Autodesk Inventor part; units mm, degrees
ref_plane "Arbeitsebene1" through (62.6214, -145.6709, 60.7697) normal (-1, 0, 0) x (0, -0.0042, 1)
ref_plane "YZ Plane" through (0, 0, 0) normal (1, 0, 0) x (0, 1, 0)
ref_plane "XZ Plane" through (0, 0, 0) normal (0, 1, 0) x (-1, 0, 0)
ref_plane "Arbeitsebene1" through (62.6214, -145.6709, 60.7697) normal (-1, 0, 0) x (0, -0.0042, 1)
sketch "Skizze1" plane through (62.6214, -145.6709, 60.7697) normal (-1, 0, 0) x (0, -0.0042, 1)
  circle A0 centre (0, 0) radius 10
  point P0 (-61.3791, 145.4152)
  dimension "d0" = 20
extrude "Extrusion1" add sketch "Skizze1" against normal blind 37
sketch "Skizze2" plane through (99.6214, -145.6709, 60.7697) normal (1, 0, 0) x (0, 0, -1)
  circle A0 centre (0, 0) radius 10
  circle A1 centre (0, 0) radius 12
  point P0 (60.7697, 145.6709)
  dimension "d3" = 24
extrude "Extrusion2" add sketch "Skizze2" along normal blind 83 contours A0 | A1
sketch "Skizze3" plane through (182.6214, -145.6709, 60.7697) normal (1, 0, 0) x (0, 0, -1)
  circle A0 centre (0, 0) radius 12
  circle A1 centre (0, 0) radius 14
  point P0 (60.7697, 145.6709)
  dimension "d6" = 28
extrude "Extrusion3" add sketch "Skizze3" along normal blind 191 contours A0 | A1
sketch "Skizze4" plane through (373.6214, -145.6709, 60.7697) normal (1, 0, 0) x (0, 0, -1)
  circle A0 centre (0, 0) radius 10
  circle A1 centre (0, 0) radius 12
  point P0 (60.7697, 145.6709)
  dimension "d9" = 24
extrude "Extrusion4" add sketch "Skizze4" along normal blind 13 contours A0 | A1
sketch "Skizze5" plane through (386.6214, -145.6709, 60.7697) normal (1, 0, 0) x (0, 0, -1)
  circle A0 centre (0, 0) radius 12
  circle A1 centre (0, 0) radius 17.5 construction
  line L0 (-8.1188, 15.5028) -> (8.1188, 15.5028)
  line L1 (8.1188, 15.5028) -> (17.5, 0)
  line L2 (17.5, 0) -> (8.1188, -15.5028)
  line L3 (8.1188, -15.5028) -> (-8.1188, -15.5028)
  line L4 (-8.1188, -15.5028) -> (-17.5, 0)
  line L5 (-17.5, 0) -> (-8.1188, 15.5028)
  point P0 (60.7697, 145.6709)
  dimension "d12" = 35
extrude "Extrusion5" add sketch "Skizze5" along normal blind 5 contours A0 | L0 L1 L2 L3 L4 L5
sketch "Skizze6" plane through (391.6214, -145.6709, 60.7697) normal (1, 0, 0) x (0, 0, -1)
  circle A0 centre (0, 0) radius 10
  circle A1 centre (0, 0) radius 12
  point P0 (60.7697, 145.6709)
  dimension "d15" = 24
extrude "Extrusion6" add sketch "Skizze6" along normal blind 10 contours A0 | A1
sketch "Skizze7" plane through (401.6214, -145.6709, 60.7697) normal (1, 0, 0) x (0, 0, -1)
  circle A0 centre (0, 0) radius 10
  circle A1 centre (0, 0) radius 10
  point P0 (60.7697, 145.6709)
  dimension "d18" = 20
extrude "Extrusion7" add sketch "Skizze7" along normal blind 40
sketch "Skizze8" plane through (62.6214, -145.6709, 60.7697) normal (-1, 0, 0) x (0, 0, 1)
  line L0 (8.1188, 15.5028) -> (17.5, 0)
  line L1 (17.5, 0) -> (8.1188, -15.5028)
  line L2 (-8.1188, 15.5028) -> (8.1188, 15.5028)
  line L3 (-17.5, 0) -> (-8.1188, 15.5028)
  line L4 (-8.1188, -15.5028) -> (-17.5, 0)
  line L5 (8.1188, -15.5028) -> (-8.1188, -15.5028)
  line L6 (13.9935, 0) -> (6.4276, 12.5028)
  line L7 (6.4276, 12.5028) -> (-6.4276, 12.5028)
  line L8 (-6.4276, 12.5028) -> (-13.9935, 0)
  line L9 (-13.9935, 0) -> (-6.4276, -12.5028)
  line L10 (-6.4276, -12.5028) -> (6.4276, -12.5028)
  line L11 (6.4276, -12.5028) -> (13.9935, 0)
  point P0 (-60.7697, 145.6709)
  dimension "d23" = 3
extrude "Extrusion8" add sketch "Skizze8" along normal blind 10 contours L11 L10 L9 L8 L7 L6
properties part number "Welle"
Part model, mm, in its own coordinate system. A direction names the side the tool comes from. Round coordinates to 2 decimals unless told otherwise and drop trailing zeros. Write each loop counter-clockwise with the first axis right and the second up, starting at its lowest first coordinate (ties: lowest second). Pieces come first, ordered by that corner, then holes. Notation, with made-up numbers: M 42,15.25 L 47,15.25 A25 ccw 47,36.25 Z; hole C 77,85 d6. An arc over 180 degrees is marked long. Return JSON: item names as keys, results as strings. Group by question number.
(1) Which spindle directions (+Z, -Z, +X, -X, +Y, -Y) get a long thin tool onto all of the face, cutting with end or side? Do faces 4 (the face through (421.34, -154.1, 55.39)), 5 (the face through (58, -158.174, 61)), 6 (the face through (99.621, -135.8, 63.5)), 7 (the face through (57.691, -151.835, 50.506)). Say none if no direction does.
(2) Saw through at C-C on x = 164.5. Write the cut outline in (y, z).
(3) Drill centre lines: probe 1 along X at (y, z) = (-133.5, 59.5); probe 2 along X at (y, z) = (-136.5, 66); probe 3 along Y at (x, z) = (364, 53.5). Where is each one in solid material? Low to high.
(4) Two-plate mould, pull along X, no slides. Class faces 1 (the face through (182.621, -139, 50)), 2 (the face through (52.621, -145, 61)), 3 (the face through (396.551, -141.075, 49.685)): +X half, -X half, draft (parallel to the pull), parting line (faces both ways), or undercut.
(5) Pin check, flat tips, straight feed: pin 1 Ø2 at (x, z) = (192, 49.5) entering from +Y; pin 2 Ø3 at (x, z) = (57.5, 62) entering from -Y; pin 3 Ø10 at (x, y) = (342, -149) entering from +Z; pin 4 Ø6 at (y, z) = (-141, 50.5) entering from +X. Stop position of each tip, or through.
Returned:
{
 "1": {"face 4": "+X", "face 5": "+Z, -Z, -X, -Y", "face 6": "none", "face 7": "-Z, -X, -Y"},
 "2": {"outline": "C -145.67,60.77 d24"},
 "3": {"probe 1": "52.62 to 62.62, 182.62 to 373.62, 386.62 to 391.62", "probe 2": "52.62 to 62.62, 99.62 to 401.62", "probe 3": "-157.64 to -133.71"},
 "4": {"face 1": "undercut", "face 2": "-X half", "face 3": "draft"},
 "5": {"pin 1": "y = -136.16", "pin 2": "y = -158.17", "pin 3": "z = 74.77", "pin 4": "x = 441.62"}
}
